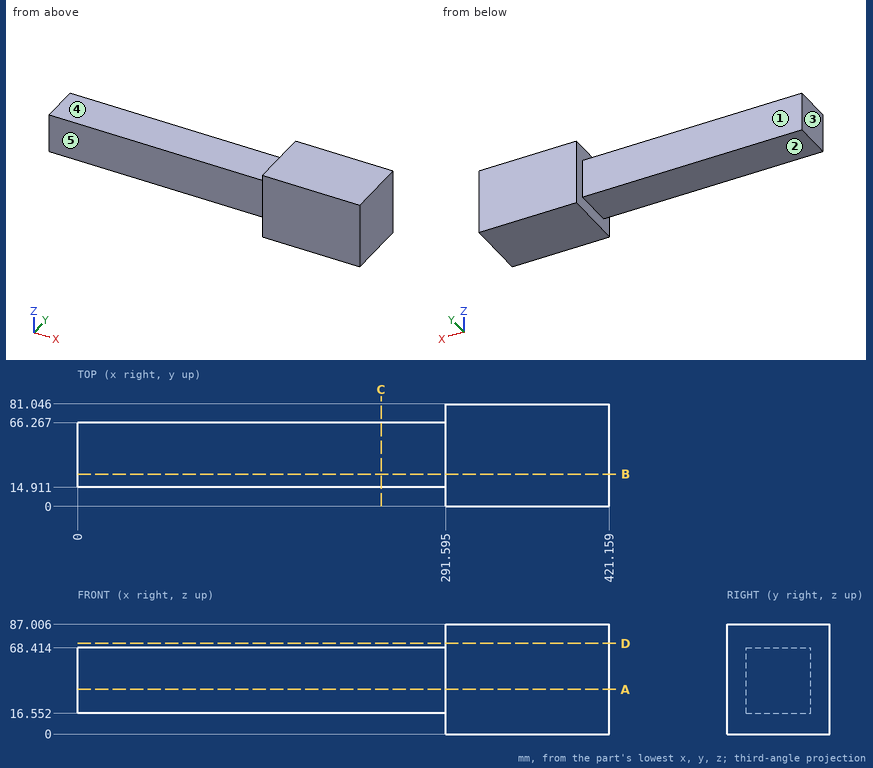
Can you work these out from the drawing? Everything is in mm from the part's minimum corner. A direction names the side the tool comes from. Give positions to 0.01 mm unless a question says otherwise; leave off trailing zeros. Order: outer loops, then holes, each group sorted by start corner. A loop starts at its lowest first (then second) coordinate and runs counter-clockwise, first axis right, second up. Notation, with made-up numbers: M 85.5,34.25 L 132.5,34.25 A30 cw 132.5,63.25 Z; hole C 20.5,-27.75 d2. An arc over 180 degrees is marked long. Use a Markdown table: item, result. Add a question column.
1. Suppose I cut it at D-D (z = 72). List the corners of the cut face in (x, y) for me (1 decimal).
2. I need wall thicknesses on probe 1 along Z at (x, y) = (185, 38.5); probe 2 along X at (y, z) = (72.5, 19) (1 decimal); probe 3 along Y at (x, z) = (268.5, 58.5). Which ranges of each line are inside material? Lowest first, please. Write a range as from..to.
3. On a 3-axis mill with a long thin cutter (end or side, diameter ignored), from which of +Z, -Z, +X, -X, +Y, -Y can I reach the whole of each face in a straight line? I mean the marked faces 1, 2, 3, 4 and 5. Say none if no direction works.
4. Suppose I cut it at C-C (x = 240.5). List the corners of the cut face in (y, z) for me.
5. Suppose I cut it at B-B (y = 25.5). List the corners of the cut face in (x, z) for me (1 decimal), and give its area (3 significant figures).
6. For pin 1 Ø4 at (x, z) = (276.5, 55) entering from -Y; pin 2 Ø8 at (x, y) = (349.5, 48) entering from -Z; pin 3 Ø2 at (x, z) = (205.5, 71) entering from +Y; pin 4 Ø1.5 at (x, z) = (231.5, 66) entering from +Y, each with a flat end and sliding along its axis, tell me the tip position at first contact or that it passes through.
7. Suppose I cut it at A-A (z = 35.5). List the corners of the cut face in (x, y) for me (1 decimal), and give its area (3 significant figures).
Results list:
| question | item | result |
|---|---|---|
| 1 | outline | M 291.6,0 L 421.2,0 L 421.2,81 L 291.6,81 Z |
| 2 | probe 1 | z = 16.55..68.41 |
| 2 | probe 2 | x = 291.6..421.2 |
| 2 | probe 3 | y = 14.91..66.27 |
| 3 | face 1 | +Z, -Z, -X, +Y |
| 3 | face 2 | -Z, -X, +Y, -Y |
| 3 | face 3 | +Z, -Z, -X, +Y, -Y |
| 3 | face 4 | +Z, -X, +Y, -Y |
| 3 | face 5 | +Z, -Z, -X, -Y |
| 4 | outline | M 14.91,16.55 L 66.27,16.55 L 66.27,68.41 L 14.91,68.41 Z |
| 5 | outline | M 0,16.6 L 291.6,16.6 L 291.6,0 L 421.2,0 L 421.2,87 L 291.6,87 L 291.6,68.4 L 0,68.4 Z |
| 5 | area | 26,400 mm² |
| 6 | pin 1 | stops at y = 14.91 |
| 6 | pin 2 | stops at z = 0 |
| 6 | pin 3 | passes through |
| 6 | pin 4 | stops at y = 66.27 |
| 7 | outline | M 0,14.9 L 291.6,14.9 L 291.6,0 L 421.2,0 L 421.2,81 L 291.6,81 L 291.6,66.3 L 0,66.3 Z |
| 7 | area | 25,500 mm² |
